Geometry check sheet. Reference: drawing and pictorial views, mm from the part's lowest x, y, z. A direction names the side the tool comes from. Give positions to 0.01 mm unless a question says otherwise; leave off trailing zeros. Order: outer loops, then holes, each group sorted by start corner. A loop starts at its lowest first (then second) coordinate and runs counter-clockwise, first axis right, second up.
Item 1: Sectioned sample at A-A on z = 19.75. Count the separate pieces of the cut face and the enclosed holes in it, and give its area (3 significant figures).
Item 2: Material ranges on line 1 along X through (y, z) = (5, 19.25) (1 decimal); line 2 along Y through (x, z) = (44, 17.95) (1 decimal); line 3 along Z through (x, y) = (6.5, 2), recorded low to high.
Item 3: Gauge pin test, flat ends, axial feed: P1, Ø5, axis at x = 5, y = 6.5, coming from the -Z side; P2, Ø1.5, axis at x = 21, y = 12.5, coming from the +Z side; P3, Ø6, axis at x = 18, y = 7, coming from the -Z side; P4, Ø1.9, axis at y = 7.5, z = 19, coming from the -X side. Record the tip position at first contact, or that the pin passes through.
Item 4: Sectioned sample at C-C on z = 15. Record the boundary of the cut face in (x, y) (1 decimal).
Item 5: Sectioned sample at D-D on y = 12.75. Record the boundary of the cut face in (x, z) (1 decimal).
Item 6: Access from +Z, -Z, +X, -X, +Y, -Y to the whole of each face (thin tool, end or side, straight path). Record for the marked faces 4, 5, 6, 7 and 8.
Item 7: Release check for a two-part mould opening along X. For the marked faces 1, 2 and 3 record: released by +X, released by -X, zero draft, split by the parting line, or undercut.
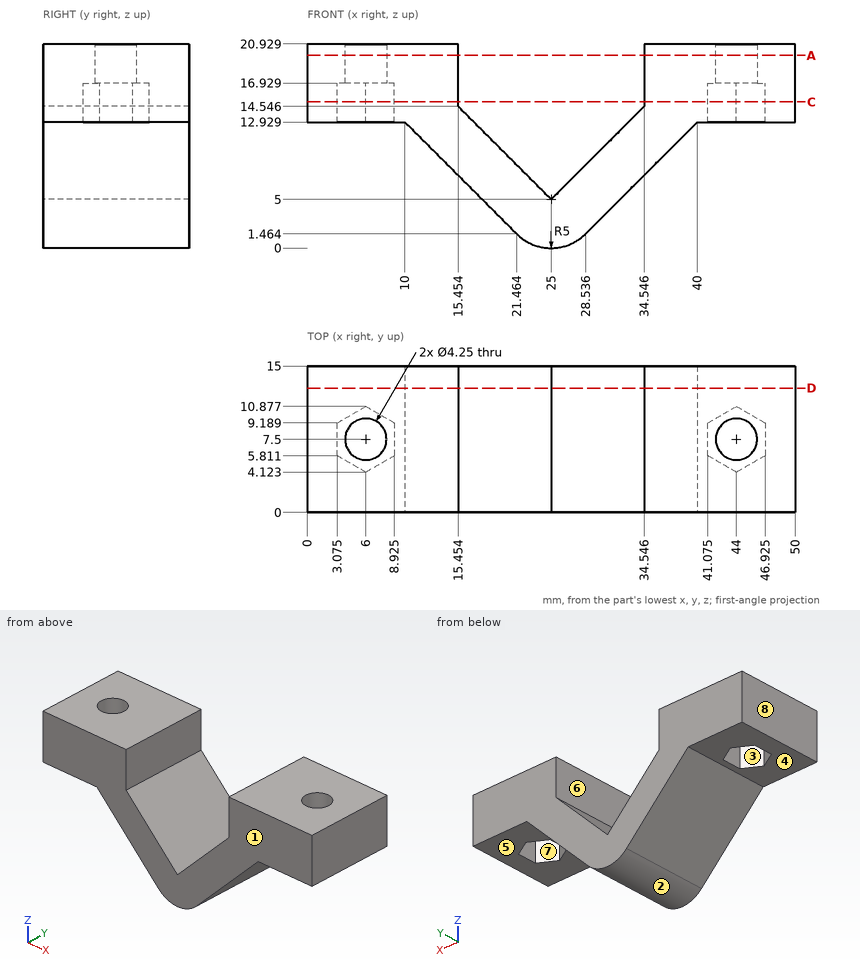
Report:
1. separate pieces: 2
1. enclosed holes: 2
1. area: 435 mm2
2. line 1: x = 0 to 15.5, 34.5 to 50
2. line 2: y = 0 to 5.4, 9.6 to 15
2. line 3: z = 12.93 to 20.93
3. P1: stops at z = 12.93
3. P2: stops at z = 9.75
3. P3: stops at z = 1.93
3. P4: stops at x = 0
4. outline: (0, 0) - (15.5, 0) - (15.5, 15) - (0, 15) - close; (34.5, 0) - (50, 0) - (50, 15) - (34.5, 15) - close; hole (3.1, 5.8) - (6, 4.1) - (8.9, 5.8) - (8.9, 9.2) - (6, 10.9) - (3.1, 9.2) - close; hole (41.1, 5.8) - (44, 4.1) - (46.9, 5.8) - (46.9, 9.2) - (44, 10.9) - (41.1, 9.2) - close
5. outline: (0, 12.9) - (10, 12.9) - (21.5, 1.5) arc R5 ccw to (28.5, 1.5) - (40, 12.9) - (50, 12.9) - (50, 20.9) - (34.5, 20.9) - (34.5, 14.5) - (25, 5) - (15.5, 14.5) - (15.5, 20.9) - (0, 20.9) - close
6. face 4: -Z, -X, +Y, -Y
6. face 5: -Z, +X, +Y, -Y
6. face 6: +Z, +Y, -Y
6. face 7: -Z
6. face 8: +Z, -Z, -X, +Y, -Y
7. face 1: zero draft
7. face 2: split by the parting line
7. face 3: undercut
